Here's how the part is built. I have some questions about the finished solid (model axes, mm). Face numbers are marked on the shaded views. A direction names the side the tool comes from. Give positions to 0.01 mm unless a question says otherwise; leave off trailing zeros. Loops run counter-clockwise (first coordinate to the right, second up) from the corner with the lowest first, then second, coordinate; pieces in that order, holes last. Notation, with made-up numbers: (24.25, 49) - (45.25, 49) arc R13 ccw to (45.25, 53) - close; hole circle Ø6 at (57.5, -26.5). An arc over 180 degrees is marked (long way). Use one line per item in the form item = value.
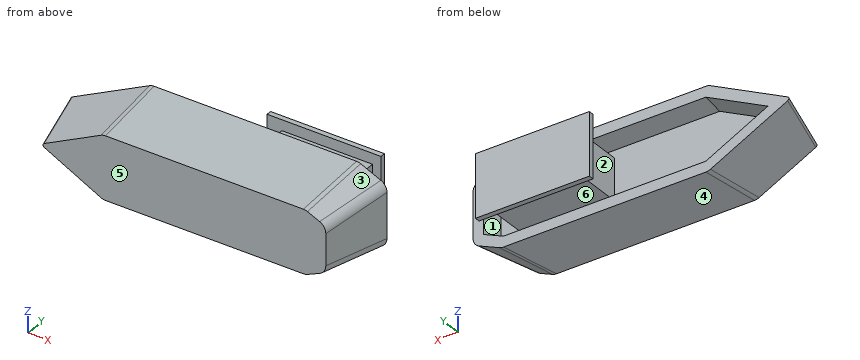
from build123d import *

# Parameters (mm, degrees)
SALIENTE_EXTRUIR1_DEPTH = 70
CHAFL_N1_SIZE           = 71.153697224
CHAFL_N1_SIZE_2         = 10
CHAFL_N2_SIZE           = 10
CHAFL_N2_SIZE_2         = 71.153697224
CHAFL_N3_SIZE           = 10
CHAFL_N3_SIZE_2         = 71.153697224
CHAFL_N4_SIZE           = 10
CHAFL_N4_SIZE_2         = 71.153697224
CHAFL_N6_SIZE           = 10
CHAFL_N6_SIZE_2         = 71.153697224
CHAFL_N7_SIZE           = 71.153697224
CHAFL_N7_SIZE_2         = 10
CHAFL_N8_SIZE           = 10
CHAFL_N8_SIZE_2         = 71.153697224
VACIADO2_DEPTH          = 20
VACIADO2_DRAFT          = -8
CROQUIS3_W              = 87.591071548
CROQUIS3_H              = 39.675716858
SALIENTE_EXTRUIR3_DEPTH = 30
CROQUIS4_W              = 110
CROQUIS4_H              = 60
SALIENTE_EXTRUIR4_DEPTH = 5
REDONDEO2_R             = 2
REDONDEO4_R             = 10
REDONDEO5_R             = 10


# Read off the part's stored shape, not the designer's step: Vaciado2
with BuildPart() as part:
    # Croquis1 → Saliente-Extruir1 (new body)
    with BuildSketch(Plane(origin=(0, 0, 0), x_dir=(1, 0, 0), z_dir=(0, 1, 0))):
        Polygon((100, -40), (-100, -40), (-180.622577483, 0), (-100, 40), (100, 40), (127.49545417, 28), (127.49545417, -28), align=None)
    extrude(amount=SALIENTE_EXTRUIR1_DEPTH)

    # Chaflán1
    # the kernel refuses this chamfer: 71.153697224, 10 mm, written as the material it takes off along each edge
    with BuildSketch(Plane(origin=(284.933017826, 0, 40), x_dir=(0, 0.999985663281603, 0.005354739139527623), z_dir=(-1, 0, 0))) as chafl_n1_piece_1:
        Polygon((CHAFL_N1_SIZE * 0.999985663279, CHAFL_N1_SIZE * 0.00535473913952), (-CHAFL_N1_SIZE_2 * 0.00535473913953, CHAFL_N1_SIZE_2 * 0.999985663282), (0, 0), align=None)
    extrude(amount=569.866035651, mode=Mode.SUBTRACT)

    # Chaflán2
    # the kernel refuses this chamfer: 71.153697224, 10 mm, written as the material it takes off along each edge
    with BuildSketch(Plane(origin=(45.508539616, 0, 112.192452367), x_dir=(0.4289599478157497, -0.26166085119417803, -0.8645964157468197), z_dir=(-0.895806416477617, 0, -0.44444444444444353))) as chafl_n2_piece_1:
        Polygon((CHAFL_N2_SIZE * 0.965159882585, -CHAFL_N2_SIZE * 0.261660851194), (-CHAFL_N2_SIZE_2 * 0.261660851194, -CHAFL_N2_SIZE_2 * 0.965159882583), (0, 0), align=None)
    extrude(amount=437.366035651, mode=Mode.SUBTRACT)

    # Chaflán3
    # the kernel refuses this chamfer: 71.153697224, 10 mm, written as the material it takes off along each edge
    with BuildSketch(Plane(origin=(-335.03676147, 0, 76.61088931), x_dir=(0.4289599478157518, -0.2616608511941785, 0.8645964157468186), z_dir=(0.895806416477616, 0, -0.4444444444444457))) as chafl_n3_piece_1:
        Polygon((CHAFL_N3_SIZE * 0.965159882585, -CHAFL_N3_SIZE * 0.261660851194), (-CHAFL_N3_SIZE_2 * 0.261660851194, -CHAFL_N3_SIZE_2 * 0.965159882583), (0, 0), align=None)
    extrude(amount=447.307518774, mode=Mode.SUBTRACT)

    # Chaflán4
    # the kernel refuses this chamfer: 71.153697224, 10 mm, written as the material it takes off along each edge
    with BuildSketch(Plane(origin=(-262.433017825, 0, -40), x_dir=(0, -0.26166085119417826, 0.9651598825854388), z_dir=(1, 0, 0))) as chafl_n4_piece_1:
        Polygon((CHAFL_N4_SIZE * 0.965159882585, -CHAFL_N4_SIZE * 0.261660851194), (-CHAFL_N4_SIZE_2 * 0.261660851194, -CHAFL_N4_SIZE_2 * 0.965159882583), (0, 0), align=None)
    extrude(amount=547.366035651, mode=Mode.SUBTRACT)

    # Chaflán6
    # the kernel refuses this chamfer: 71.153697224, 10 mm, written as the material it takes off along each edge
    with BuildSketch(Plane(origin=(-46.581032062, 0, -103.97320713), x_dir=(-0.3860639530341748, -0.2616608511941783, 0.8845836439364931), z_dir=(0.9165151389911683, 0, 0.3999999999999993))) as chafl_n6_piece_1:
        Polygon((CHAFL_N6_SIZE * 0.965159882585, -CHAFL_N6_SIZE * 0.261660851194), (-CHAFL_N6_SIZE_2 * 0.261660851194, -CHAFL_N6_SIZE_2 * 0.965159882583), (0, 0), align=None)
    extrude(amount=374.866035651, mode=Mode.SUBTRACT)

    # Chaflán7
    # the kernel refuses this chamfer: 71.153697224, 10 mm, written as the material it takes off along each edge
    with BuildSketch(Plane(origin=(296.989364706, 0, -45.97320713), x_dir=(0.002141895655810909, 0.999985663281603, 0.004907699486725296), z_dir=(-0.9165151389911683, 0, 0.3999999999999993))) as chafl_n7_piece_1:
        Polygon((CHAFL_N7_SIZE * 0.999985663279, CHAFL_N7_SIZE * 0.00535473913952), (-CHAFL_N7_SIZE_2 * 0.00535473913953, CHAFL_N7_SIZE_2 * 0.999985663282), (0, 0), align=None)
    extrude(amount=374.866035651, mode=Mode.SUBTRACT)

    # Chaflán8
    # the kernel refuses this chamfer: 71.153697224, 10 mm, written as the material it takes off along each edge
    with BuildSketch(Plane(origin=(127.49545417, 0, -202.022123314), x_dir=(-0.9651598825854388, -0.26166085119417826, 0), z_dir=(0, 0, 1))) as chafl_n8_piece_1:
        Polygon((CHAFL_N8_SIZE * 0.965159882585, -CHAFL_N8_SIZE * 0.261660851194), (-CHAFL_N8_SIZE_2 * 0.261660851194, -CHAFL_N8_SIZE_2 * 0.965159882583), (0, 0), align=None)
    extrude(amount=404.044246628, mode=Mode.SUBTRACT)


with BuildPart() as vaciado2_tool:
    # Vaciado2 outline → Vaciado2 (with draft: the straight prism first)
    with BuildSketch(Plane(origin=(0, 50, 0), x_dir=(1, 0, 0), z_dir=(0, 1, 0))):
        Polygon((114.42422018, 19.442868688), (97.271874618, 26.92876601), (-96.935637901, 26.92876601), (-151.212301005, 0), (-96.935637901, -26.92876601), (97.271874618, -26.92876601), (114.42422018, -19.442868688), align=None)
    extrude(amount=VACIADO2_DEPTH)
    # Vaciado2: the draft: its side faces are tilted about the plane it starts from
    vaciado2_sides = [vaciado2_tool.faces().sort_by_distance(p)[0] for p in [
        (105.848047399, 60, -23.185817349),
        (0.168118358, 60, -26.92876601),
        (-124.073969453, 60, -13.464383005),
        (-124.073969453, 60, 13.464383005),
        (0.168118358, 60, 26.92876601),
        (105.848047399, 60, 23.185817349),
        (114.42422018, 60, 0),
    ]]
    draft(vaciado2_sides, Plane(origin=(0, 50, 0), x_dir=(1, 0, 0), z_dir=(0, 1, 0)), VACIADO2_DRAFT)


with BuildPart() as part_1:
    add(part.part)

    # Vaciado2: cut by vaciado2_tool
    add(vaciado2_tool.part, mode=Mode.SUBTRACT)

    # Croquis3 → Saliente-Extruir3 (add, symmetric)
    with BuildSketch(Plane(origin=(0, 70, 0), x_dir=(1, 0, 0), z_dir=(0, 1, 0))):
        with Locations((48.537776825, 0)):
            Rectangle(CROQUIS3_W, CROQUIS3_H)
    extrude(amount=SALIENTE_EXTRUIR3_DEPTH, both=True)

    # Croquis4 → Saliente-Extruir4 (add)
    with BuildSketch(Plane(origin=(0, 100, 0), x_dir=(1, 0, 0), z_dir=(0, 1, 0))):
        with Locations((45.333312599, 0)):
            Rectangle(CROQUIS4_W, CROQUIS4_H)
    extrude(amount=SALIENTE_EXTRUIR4_DEPTH)

    # Redondeo2
    redondeo2_edges = [part_1.edges().sort_by_distance(p)[0] for p in [
        (-169.190168216, 35, 0),
    ]]
    fillet(redondeo2_edges, radius=REDONDEO2_R)

    # Redondeo4
    redondeo4_edges = [part_1.edges().sort_by_distance(p)[0] for p in [
        (98.939518779, 35, -34.918929215),
        (98.939518779, 35, 34.918929215),
        (122.414383384, 35, -24.673658359),
        (122.414383384, 35, 24.673658359),
    ]]
    fillet(redondeo4_edges, radius=REDONDEO4_R)

    # Redondeo5
    redondeo5_edges = [part_1.edges().sort_by_distance(p)[0] for p in [
        (-98.80881631, 35, 34.918929215),
        (-98.80881631, 35, -34.918929215),
    ]]
    fillet(redondeo5_edges, radius=REDONDEO5_R)


solid = part_1.part
(1) For P1, Ø12, axis at y = 28, z = 30, coming from the +X side; P2, Ø5.5, axis at y = 101.5, z = 6.5, coming from the +X side; P3, Ø15, axis at x = 43, y = 80, coming from the +Z side, each with a flat end and sliding along its axis, tell me the tip position at first contact or that it passes through.
Geometry says:
P1 = 119.21
P2 = 100.33
P3 = 19.84
(2) If we section it at D-D (y = 83.5): List the corners of the cut face in (x, z) for me.
Geometry says:
outline = (4.74, -19.84) - (92.33, -19.84) - (92.33, 19.84) - (4.74, 19.84) - close
(3) Thinking about a two-plate mould opening in Z: for the marked faces 4, 5 and 6, which applies, pulls with the +Z half, pulls with the -Z half, needs draft (parallel to the pull), parting line crosses it, or undercut?
Geometry says:
face_4 = pulls with the -Z half
face_5 = needs draft
face_6 = undercut
(4) If we section it at A-A (x = -74): List the corners of the cut face in (y, z) for me.
Geometry says:
outline = (0, -30) - (70, -39.84) - (70, -29.74) - (50, -26.93) - (50, 26.93) - (70, 29.74) - (70, 39.84) - (0, 30) - close
(5) If I drill on probe 1 along Y at (x, z) = (84.5, -20.5); probe 2 along X at (y, z) = (61.5, -19.5); probe 3 along X at (y, z) = (64, -4.5), over which ranges is the centre line in solid material (lowest first)?
Geometry says:
probe_1 = 0 to 50, 100 to 105
probe_2 = -138.27 to -115.55, 4.74 to 92.33, 116.04 to 126.14
probe_3 = -169.29 to -146.57, 4.74 to 92.33, 116.39 to 126.49
(6) If we section it at B-B (y = 55.5): Give the number of separate pieces and of enclosed holes in the cut face, plus the area to 3 significant figures.
Geometry says:
separate_pieces = 2
enclosed_holes = 1
area = 9,870 mm²
(7) If we section it at C-C (z = -4.5): List the corners of the cut face in (x, y) for me, plus the area to 3 significant figures.
Geometry says:
outline = (-171.19, 70) - (-149.05, 0) - (117.5, 0) - (127.33, 70) - (117.24, 70) - (114.42, 50) - (92.33, 50) - (92.33, 100) - (100.33, 100) - (100.33, 105) - (-9.67, 105) - (-9.67, 100) - (4.74, 100) - (4.74, 50) - (-142.14, 50) - (-148.47, 70) - close
area = 19,500 mm²
(8) For the marked faces 1, 2 and 3, which set-ups out of +Z, -Z, +X, -X, +Y, -Y let a thin tool reach every point of the face, with its end or its side?
Geometry says:
face_1 = +Y
face_2 = none
face_3 = +Z, +X, -Y
